Solid Edge part; units mm, degrees
sketch "Sketch1" plane through (0, 0, 0) normal (0, 0, 1) x (1, 0, 0)
  line L0 (25, -40) -> (25, 40)
  line L1 (25, 40) -> (-25, 40)
  line L2 (-25, 40) -> (-25, -40)
  line L3 (-25, -40) -> (25, -40)
extrude "Protrusion1" add sketch "Sketch1" against normal blind 12
sketch "Sketch2" plane through (0, 0, -12) normal (0, 0, -1) x (0, -1, 0)
  line L0 (-40, -25) -> (-40, 25)
  line L1 (-40, 25) -> (-28, 25)
  line L2 (-28, 25) -> (-28, -25)
  line L3 (-28, -25) -> (-40, -25)
extrude "ExtrudedProtrusion_2" add sketch "Sketch2" along normal blind 70
sketch "Sketch3" plane through (0, -6, -12) normal (0, 0, -1) x (0, -1, 0)
  line L0 (34, 6) -> (-34, 6)
  line L1 (-34, 6) -> (-34, -6)
  line L2 (-34, -6) -> (34, -6)
  line L3 (34, -6) -> (34, 6)
  dimension "D1" = 34
extrude "ExtrudedProtrusion_3" add sketch "Sketch3" along normal blind 50
hole "Hole_1" at (-13.5209, 40, -70) direction (0, -1, 0) diameter 6 end up to next
hole "Hole1" at (13.5209, 40, -70) direction (0, -1, 0) diameter 6 end up to next
Part model, mm, in its own coordinate system. A direction names the side the tool comes from. Coordinates: 2 decimals unless noted, no trailing zeros. Order: outer loops, then holes, each group sorted by start corner. A loop starts at its lowest first (then second) coordinate and runs counter-clockwise, first axis right, second up. Notation, with made-up numbers: M -35.75,12.25 L 6.25,12.25 A22 cw 6.25,30.25 Z; hole C 47.25,31 d4. An arc over 180 degrees is marked long. Use a Markdown table: item, result.
(1) Cut at B-B on x = -12.5. Write the cut outline in (y, z), then the cut area to 3 significant figures.
A:
| item | result |
|---|---|
| outline | M -40,-12 L 28,-12 L 28,-67.18 L 40,-67.18 L 40,0 L -40,0 Z; M 28,-82 L 40,-82 L 40,-72.82 L 28,-72.82 Z |
| area | 1,730 mm^2 |
(2) Cut at C-C on y = 0.5. Write the cut outline in (x, z).
A:
| item | result |
|---|---|
| outline | M -25,-12 L -6,-12 L -6,-62 L 6,-62 L 6,-12 L 25,-12 L 25,0 L -25,0 Z |
(3) Cut at A-A on z = -70. Write the cut outline in (x, y).
A:
| item | result |
|---|---|
| outline | M -25,28 L -16.52,28 L -16.52,40 L -25,40 Z; M -10.52,28 L 10.52,28 L 10.52,40 L -10.52,40 Z; M 16.52,28 L 25,28 L 25,40 L 16.52,40 Z |
(4) Flat gauge pins, fed straight in: pin 1 (15 mm diameter, centred on y = -19.5, z = -33.5, fed in from -X); pin 2 (12 mm diameter, centred on y = -25, z = -31, fed in from +X); pin 3 (9.5 mm diameter, centred on x = 13.52, z = -70, fed in from +Y); pin 4 (5.5 mm diameter, centred on x = -20, y = -9, fed in from -Z). Where does each tip first touch, or does it go through?
A:
| item | result |
|---|---|
| pin 1 | stops at x = -6 |
| pin 2 | stops at x = 6 |
| pin 3 | stops at y = 40 |
| pin 4 | stops at z = -12 |
(5) Pull direction X, two halves, no side cores. Call faces 6 (the flat face through (0, -40, -24)), 7 (the flat face through (6, -6, -37)), 8 (the cylindrical face through (-11.49, 34.08, -72.21)): released by +X, released by -X, zero draft, split by the parting line, or undercut.
A:
| item | result |
|---|---|
| face 6 | zero draft |
| face 7 | released by +X |
| face 8 | undercut |
(6) Tool access for faces 1 (the flat face through (0, 34, -82)), 2 (the flat face through (0, 40, -40)), 3 (the flat face through (-16, -6, -12)), 4 (the flat face through (0, -6, -62)), 5 (the flat face through (15, -6, -12)): list every direction of +Z, -Z, +X, -X, +Y, -Y with a clear straight run to the whole face (end or side of a thin tool).
A:
| item | result |
|---|---|
| face 1 | -Z, +X, -X, +Y, -Y |
| face 2 | +Z, -Z, +X, -X, +Y |
| face 3 | -Z, -X, -Y |
| face 4 | -Z, +X, -X, -Y |
| face 5 | -Z, +X, -Y |
(7) Cut at D-D on x = -1. Write the cut outline in (y, z), then the cut area to 3 significant figures.
A:
| item | result |
|---|---|
| outline | M -40,-62 L 28,-62 L 28,-82 L 40,-82 L 40,0 L -40,0 Z |
| area | 5,200 mm^2 |
(8) Probe L1, parallel to X at y = 36.5, z = -70; L2, parallel to X at y = 20, z = -43; L3, parallel to Z at x = -19.5, y = -4. List the from-to ranges inside material, lowest first.
A:
| item | result |
|---|---|
| L1 | x = -25 to -16.52, -10.52 to 10.52, 16.52 to 25 |
| L2 | x = -6 to 6 |
| L3 | z = -12 to 0 |
